Drawing for the job (mm, zero at the part's lowest x, y, z). A direction names the side the tool comes from. Round coordinates to 2 decimals unless told otherwise and drop trailing zeros. Write each loop counter-clockwise with the first axis right and the second up, starting at its lowest first coordinate (ties: lowest second). Pieces come first, ordered by that corner, then holes. Notation, with made-up numbers: M 6,-30 L 57,-30 A22 ccw 57,8 Z; hole C 61.25,82.5 d10. An arc over 180 degrees is marked long. Use a Markdown table: item, result.
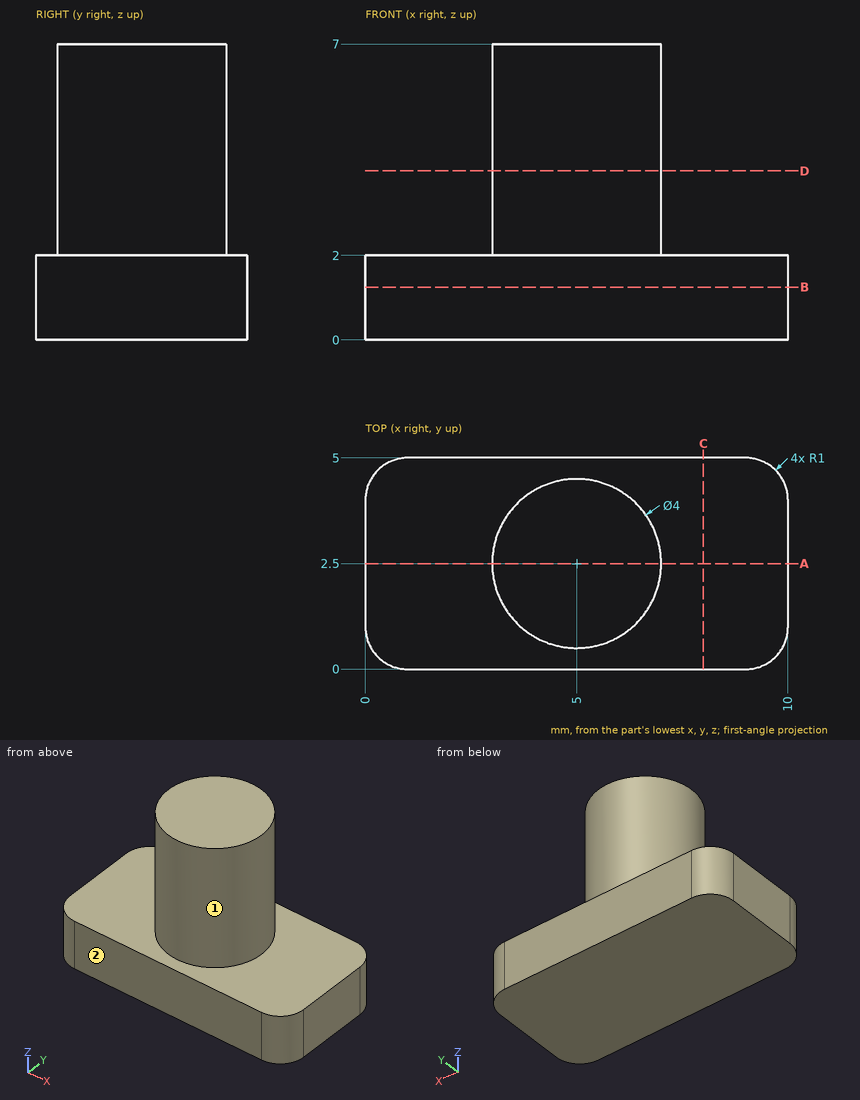
Q1. Cut at D-D on z = 4. Give the cut face in (x, y).
Response values:
| item | result |
|---|---|
| outline | C 5,2.5 d4 |
Q2. Cut at B-B on z = 1.25. Give the cut face in (x, y).
Response values:
| item | result |
|---|---|
| outline | M 0,1 A1 ccw 1,0 L 9,0 A1 ccw 10,1 L 10,4 A1 ccw 9,5 L 1,5 A1 ccw 0,4 Z |
Q3. Cut at A-A on y = 2.5. Give the cut face in (x, z).
Response values:
| item | result |
|---|---|
| outline | M 0,0 L 10,0 L 10,2 L 7,2 L 7,7 L 3,7 L 3,2 L 0,2 Z |
Q4. Drop a flat-ended pin along its axis: P1, Ø1, axis at x = 1, y = 1, coming from the +Z side. Give the stop position or say it passes through.
Response values:
| item | result |
|---|---|
| P1 | stops at z = 2 |
Q5. Cut at C-C on x = 8. Give the cut face in (y, z), and give its area (3 significant figures).
Response values:
| item | result |
|---|---|
| outline | M 0,0 L 5,0 L 5,2 L 0,2 Z |
| area | 10.0 mm2 |
Q6. Drill centre lines: L1, parallel to Z at x = 3, y = 1.05; L2, parallel to X at y = 3.5, z = 3.25; L3, parallel to X at y = 3.9, z = 5.25. Where is each one in solid material? Low to high.
Response values:
| item | result |
|---|---|
| L1 | z = 0 to 2 |
| L2 | x = 3.27 to 6.73 |
| L3 | x = 3.57 to 6.43 |
Q7. Which spindle directions (+Z, -Z, +X, -X, +Y, -Y) get a long thin tool onto all of the face, cutting with end or side? Do the marked faces 1 and 2. Say none if no direction does.
Response values:
| item | result |
|---|---|
| face 1 | +Z |
| face 2 | +Z, -Z, +X, -X, -Y |
